Design review of the part built by this model. Coordinates are the model's own, in mm. Face numbers are marked on the shaded views. A direction names the side the tool comes from. Coordinates: 2 decimals unless noted, no trailing zeros. Write each loop counter-clockwise with the first axis right and the second up, starting at its lowest first coordinate (ties: lowest second). Pieces come first, ordered by that corner, then holes.
```python
from build123d import *

# Parameters (mm, degrees)
F0_W     = 88.720875
F0_H     = 30
F1_DEPTH = 70
F2_R     = 7.5
F3_DEPTH = 25


with BuildPart() as f1:
    # F0 (on Right) → F1 (new body)
    with BuildSketch(Plane.YZ):
        with Locations((59.895014, 15)):
            Rectangle(F0_W, F0_H)
        Polygon((0, 94.020176), (0, 0), (15.534577, 0), (15.534577, 30), (15.534577, 94.020176), align=None)
    extrude(amount=F1_DEPTH)

    # F2 (on face) → F3 (cut)
    with BuildSketch(Plane.XZ):
        with Locations((35, 71.520176)):
            Circle(F2_R)
    extrude(amount=-F3_DEPTH, mode=Mode.SUBTRACT)


solid = f1.part
```
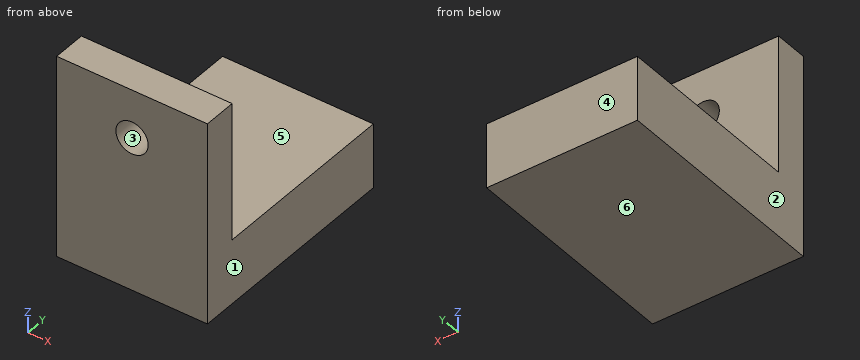
(1) Consider section D-D (y = 79). Give the boundary of the cut face in (x, z).
(2) Consider section B-B (z = 81.5). Give the boundary of the cut face in (x, y).
(3) Insertion check: pin 1 Ø4 at (x, y) = (17.5, 54) entering from +Z; pin 2 Ø4 at (x, z) = (47, 54) entering from +Y; pin 3 Ø12 at (x, z) = (35, 71.52) entering from +Y; pin 4 Ø4 at (y, z) = (17.5, 70.5) entering from +X. Each pin has a flat end and moves straight along its axis. Give the tip position at first contact, or say it passes through.
(4) Consider section C-C (y = 11.5). Give the boundary of the cut face in (x, z).
(5) For the marked faces 5 and 6, list the 3-axis set-ups (+Z, -Z, +X, -X, +Y, -Y) from which the entire face can be reached by the end or side of a thin tool; tool diameter is ignored.
(6) Consider section A-A (x = 35). Give the boundary of the cut face in (y, z).
(7) Mouldability with a two-part tool opening along X and no side actions: class the marked faces 1, 2, 3 and 4 as +X half, -X half, draft (parallel to the pull), parting line (faces both ways), or undercut.
(8) Wall thickness on line 1 (Y direction, x = 60, z = 31.5); line 2 (Z direction, x = 15, y = 31.5); line 3 (Z direction, x = 35, y = 9.25): over which ranges is each line inside the solid? List them lowest first.
Results:
1. outline: (0, 0) - (70, 0) - (70, 30) - (0, 30) - close
2. outline: (0, 0) - (70, 0) - (70, 15.53) - (0, 15.53) - close
3. pin 1: stops at z = 30
3. pin 2: stops at y = 15.53
3. pin 3: passes through
3. pin 4: stops at x = 70
4. outline: (0, 0) - (70, 0) - (70, 94.02) - (0, 94.02) - close; hole circle Ø15 at (35, 71.52)
5. face 5: +Z, +X, -X, +Y
5. face 6: -Z, +X, -X, +Y, -Y
6. outline: (0, 0) - (104.26, 0) - (104.26, 30) - (15.53, 30) - (15.53, 64.02) - (0, 64.02) - close; (0, 79.02) - (15.53, 79.02) - (15.53, 94.02) - (0, 94.02) - close
7. face 1: +X half
7. face 2: -X half
7. face 3: undercut
7. face 4: draft
8. line 1: y = 0 to 15.53
8. line 2: z = 0 to 30
8. line 3: z = 0 to 64.02, 79.02 to 94.02
